For this review, take the finished solid that the model builds, in its own axes (mm). A direction names the side the tool comes from. Coordinates: 2 decimals unless noted, no trailing zeros. Order: outer loops, then holes, each group sorted by start corner. A loop starts at its lowest first (then second) coordinate and runs counter-clockwise, first axis right, second up. Notation, with made-up numbers: M -35.5,64 L 21.5,64 A18 cw 21.5,79 Z; hole C 41,86 d1. An arc over 180 degrees is marked long. Use one line per item in the form item = value. Start each with the question number.
```python
from build123d import *

# Parameters (mm, degrees)
ESQUISSE1_R        = 13.5
ESQUISSE1_R_2      = 5
ESQUISSE1_R_3      = 10
ESQUISSE1_R_4      = 2
BOSS_EXTRU_1_DEPTH = 6


with BuildPart() as part:
    # Esquisse1 → Boss.-Extru.1 (new body)
    with BuildSketch(Plane(origin=(0, 0, 0), x_dir=(1, 0, 0), z_dir=(0, 1, 0))):
        with BuildLine():
            Line((-160, 25), (-77.459666924, 25))
            ThreePointArc((-77.459666924, 25), (-63.694722892, 28.344300501), (-52.998719474, 37.631578947))
            ThreePointArc((-52.998719474, 37.631578947), (0, 65), (52.998719474, 37.631578947))
            ThreePointArc((52.998719474, 37.631578947), (63.694722892, 28.344300501), (77.459666924, 25))
            Line((77.459666924, 25), (160, 25))
            ThreePointArc((160, 25), (170.606601718, 20.606601718), (175, 10))
            Line((175, 10), (175, -10))
            ThreePointArc((175, -10), (170.606601718, -20.606601718), (160, -25))
            Line((160, -25), (77.459666924, -25))
            ThreePointArc((77.459666924, -25), (63.694722892, -28.344300501), (52.998719474, -37.631578947))
            ThreePointArc((52.998719474, -37.631578947), (0, -65), (-52.998719474, -37.631578947))
            ThreePointArc((-52.998719474, -37.631578947), (-63.694722892, -28.344300501), (-77.459666924, -25))
            Line((-77.459666924, -25), (-160, -25))
            ThreePointArc((-160, -25), (-170.606601718, -20.606601718), (-175, -10))
            Line((-175, -10), (-175, 10))
            ThreePointArc((-175, 10), (-170.606601718, 20.606601718), (-160, 25))
        make_face()
        Circle(ESQUISSE1_R, mode=Mode.SUBTRACT)
        with Locations((-115, 0)):
            Circle(ESQUISSE1_R_2, mode=Mode.SUBTRACT)
        with Locations((-155, 0)):
            Circle(ESQUISSE1_R_2, mode=Mode.SUBTRACT)
        with Locations((155, 0)):
            Circle(ESQUISSE1_R_2, mode=Mode.SUBTRACT)
        with Locations((115, 0)):
            Circle(ESQUISSE1_R_2, mode=Mode.SUBTRACT)
        with Locations((85, 0)):
            Circle(ESQUISSE1_R_3, mode=Mode.SUBTRACT)
        with Locations((-25, 0)):
            Circle(ESQUISSE1_R_4, mode=Mode.SUBTRACT)
        with Locations((25, 0)):
            Circle(ESQUISSE1_R_4, mode=Mode.SUBTRACT)
        with Locations((77, 17.5)):
            Circle(ESQUISSE1_R_4, mode=Mode.SUBTRACT)
        with Locations((77, -17.5)):
            Circle(ESQUISSE1_R_4, mode=Mode.SUBTRACT)
    extrude(amount=BOSS_EXTRU_1_DEPTH)


solid = part.part
```
1. Consider section B-B, the plane x = 0. Write out the cut boundary in (y, z), plus the area to 3 significant figures.
2. Consider section D-D, the plane z = -57. Write out the cut boundary in (x, y).
3. Consider section A-A, the plane y = 1.1. Give the number of separate pieces and of enclosed holes in the cut face, plus the area to 3 significant figures.
4. To check wall thickness, follow line 1 (X direction, y = 0.4, z = -9); line 2 (X direction, y = 2.3, z = 16); line 3 (Z direction, x = 97, y = 2.2). State the ranges of each line that lie inside material, in increasing order.
5. For pin 1 Ø2 at (x, y) = (139.5, 3) entering from +Z; pin 2 Ø3.5 at (x, z) = (77, -17.5) entering from -Y; pin 3 Ø1.8 at (x, y) = (-116, 4) entering from -Z, all flat-tipped, find the tip position at first contact; note any pin that passes through.
6. The part is to be moulded in two halves that separate along Z. For faces 6 (the cylindrical face through (170.72, 2.96, 20.49)), 7 (the flat face through (175, 3, 0)), 8 (the cylindrical face through (150, 3, 0)), 9 (the cylindrical face through (-110.381, 2.958, 1.915)), say which applies: pulls with the +Z half, pulls with the -Z half, needs draft (parallel to the pull), parting line crosses it, or undercut.
7. Tool access review of faces 1 (the flat face through (-119, 3, -25)), 2 (the cylindrical face through (-0.868, 2.958, -64.994)), 3 (the cylindrical face through (0.868, 2.958, 64.994)), 4 (the flat face through (118, 3, -25)), 5 (the flat face through (-118, 3, 25)): name each direction out of +Z, -Z, +X, -X, +Y, -Y from which nothing blocks a thin tool from reaching the whole face with its end or side.
8. Consider section C-C, the plane x = 115. Write out the cut boundary in (y, z).
Answers follow:
q1.outline = M 0,-65 L 6,-65 L 6,-13.5 L 0,-13.5 Z; M 0,13.5 L 6,13.5 L 6,65 L 0,65 Z
q1.area = 618 mm²
q2.outline = M -31.24,0 L 31.24,0 L 31.24,6 L -31.24,6 Z
q3.separate_pieces = 1
q3.enclosed_holes = 10
q3.area = 23,200 mm²
q4.line_1 = -175 to -10.06, 10.06 to 80.64, 89.36 to 175
q4.line_2 = -173.75 to 75.68, 78.32 to 173.75
q4.line_3 = -25 to 25
q5.pin_1 = 25
q5.pin_2 = through
q5.pin_3 = -25
q6.face_6 = pulls with the +Z half
q6.face_7 = needs draft
q6.face_8 = undercut
q6.face_9 = undercut
q7.face_1 = -Z, -X, +Y, -Y
q7.face_2 = -Z, +Y, -Y
q7.face_3 = +Z, +Y, -Y
q7.face_4 = -Z, +X, +Y, -Y
q7.face_5 = +Z, -X, +Y, -Y
q8.outline = M 0,-25 L 6,-25 L 6,-5 L 0,-5 Z; M 0,5 L 6,5 L 6,25 L 0,25 Z
